```python
from build123d import *

# Parameters (mm, degrees)
SKETCH2_W           = 200
SKETCH2_H           = 95
BOSS_EXTRUDE1_DEPTH = 11
SKETCH3_W           = 200
SKETCH3_H           = 95
BOSS_EXTRUDE2_DEPTH = 2
SKETCH4_W           = 22
SKETCH4_H           = 35
SKETCH4_W_2         = 10
SKETCH4_H_2         = 26.5
SKETCH4_W_3         = 3
SKETCH4_H_3         = 8
SKETCH4_W_4         = 15
SKETCH4_H_4         = 15
BOSS_EXTRUDE3_DEPTH = 5
CUT_EXTRUDE1_DEPTH  = 7
SKETCH9_W           = 10
SKETCH9_H           = 3
BOSS_EXTRUDE4_DEPTH = 11
SKETCH7_W           = 220
SKETCH7_H           = 95
BOSS_EXTRUDE5_DEPTH = 2
FILLET1_R           = 2
FILLET2_R           = 2
SKETCH10_R          = 2.1
CUT_EXTRUDE2_DEPTH  = 6


with BuildPart() as part:
    # Sketch2 → Boss-Extrude1 (new body)
    with BuildSketch(Plane(origin=(0, 0, 0), x_dir=(1, 0, 0), z_dir=(0, 1, 0))):
        Rectangle(SKETCH2_W, SKETCH2_H)
        Polygon((21.5, 4.091136268), (21.5, 45), (93.5, 45), (93.5, -45), (21.5, -45), (21.5, -5.908863732), (10, -5.908863732), (10, -11), (-10, -31), (-71.5, -31), (-71.5, -41), (-93.5, -41), (-93.5, 41), (-71.5, 41), (-71.5, -16), (-10, -16), (-10, 8.5), (-19, 8.5), (-19, 43.5), (-10, 43.5), (-10, 46.5), (10, 46.5), (10, 43.5), (19, 43.5), (19, 8.5), (10, 8.5), (10, 4.091136268), align=None, mode=Mode.SUBTRACT)
    extrude(amount=BOSS_EXTRUDE1_DEPTH)

    # Sketch3 → Boss-Extrude2 (add)
    with BuildSketch(Plane.XZ):
        Rectangle(SKETCH3_W, SKETCH3_H)
    extrude(amount=BOSS_EXTRUDE2_DEPTH)

    # Sketch4 → Boss-Extrude3 (add)
    with BuildSketch(Plane(origin=(0, 0, 0), x_dir=(1, 0, 0), z_dir=(0, 1, 0))):
        with Locations((-82.5, 23.5)):
            Rectangle(SKETCH4_W, SKETCH4_H)
        with Locations((-0.04618168, 33.25)):
            Rectangle(SKETCH4_W_2, SKETCH4_H_2)
        with Locations((-92, -37)):
            Rectangle(SKETCH4_W_3, SKETCH4_H_3)
        with Locations((29, 37.5)):
            Rectangle(SKETCH4_W_4, SKETCH4_H_4)
        with Locations((86, 37.5)):
            Rectangle(SKETCH4_W_4, SKETCH4_H_4)
        with Locations((86, -37.5)):
            Rectangle(SKETCH4_W_4, SKETCH4_H_4)
        with Locations((29, -37.5)):
            Rectangle(SKETCH4_W_4, SKETCH4_H_4)
    extrude(amount=BOSS_EXTRUDE3_DEPTH)

    # Sketch5 → Cut-Extrude1 (cut)
    with BuildSketch(Plane.XY.offset(-46.5)):
        with BuildLine():
            Line((-2.94618168, 9.6), (2.85381832, 9.6))
            ThreePointArc((2.85381832, 9.6), (4.60381832, 7.85), (2.85381832, 6.1))
            Line((2.85381832, 6.1), (-2.94618168, 6.1))
            ThreePointArc((-2.94618168, 6.1), (-4.69618168, 7.85), (-2.94618168, 9.6))
        make_face()
    extrude(amount=-CUT_EXTRUDE1_DEPTH, mode=Mode.SUBTRACT)

    # Sketch9 → Boss-Extrude4 (add)
    with BuildSketch(Plane(origin=(0, 0, 0), x_dir=(1, 0, 0), z_dir=(0, 1, 0))):
        with Locations((-0.04618168, 18.5)):
            Rectangle(SKETCH9_W, SKETCH9_H)
    extrude(amount=BOSS_EXTRUDE4_DEPTH)

    # Sketch7 → Boss-Extrude5 (add)
    with BuildSketch(Plane.XZ.offset(2)):
        Rectangle(SKETCH7_W, SKETCH7_H)
    extrude(amount=-BOSS_EXTRUDE5_DEPTH)

    # Fillet1
    fillet1_edges = [part.edges().sort_by_distance(p)[0] for p in [
        (100, 0, 0),
        (-100, 0, 0),
    ]]
    fillet(fillet1_edges, radius=FILLET1_R)

    # Fillet2
    fillet2_edges = [part.edges().sort_by_distance(p)[0] for p in [
        (10, 5.5, -43.5),
        (-10, 5.5, -43.5),
        (-19, 5.5, -43.5),
        (-19, 5.5, -8.5),
        (-10, 5.5, -8.5),
        (-10, 5.5, 16),
        (-71.5, 5.5, 16),
        (-71.5, 5.5, 31),
        (-10, 5.5, 31),
        (10, 5.5, 11),
        (10, 5.5, 5.908863732),
        (21.5, 5.5, 5.908863732),
        (21.5, 5.5, -4.091136268),
        (10, 5.5, -4.091136268),
        (10, 5.5, -8.5),
        (19, 5.5, -8.5),
        (19, 5.5, -43.5),
    ]]
    fillet(fillet2_edges, radius=FILLET2_R)

    # Sketch10 → Cut-Extrude2 (cut)
    with BuildSketch(Plane(origin=(0, 11, 0), x_dir=(1, 0, 0), z_dir=(0, 1, 0))):
        with Locations(Location((-96, -43.5, 0), (0, 0, 270))):
            Circle(SKETCH10_R)
        with Locations(Location((-5, -43.5, 0), (0, 0, 270))):
            Circle(SKETCH10_R)
        with Locations(Location((5, -43.5, 0), (0, 0, 270))):
            Circle(SKETCH10_R)
        with Locations(Location((97, -43.5, 0), (0, 0, 270))):
            Circle(SKETCH10_R)
        with Locations(Location((97, 43.5, 0), (0, 0, 270))):
            Circle(SKETCH10_R)
        with Locations(Location((-26.428932188, 43.5, 0), (0, 0, 270))):
            Circle(SKETCH10_R)
        with Locations(Location((-36.428932188, 43.5, 0), (0, 0, 270))):
            Circle(SKETCH10_R)
        with Locations(Location((-96, 43.5, 0), (0, 0, 270))):
            Circle(SKETCH10_R)
    extrude(amount=-CUT_EXTRUDE2_DEPTH, mode=Mode.SUBTRACT)


solid = part.part
```
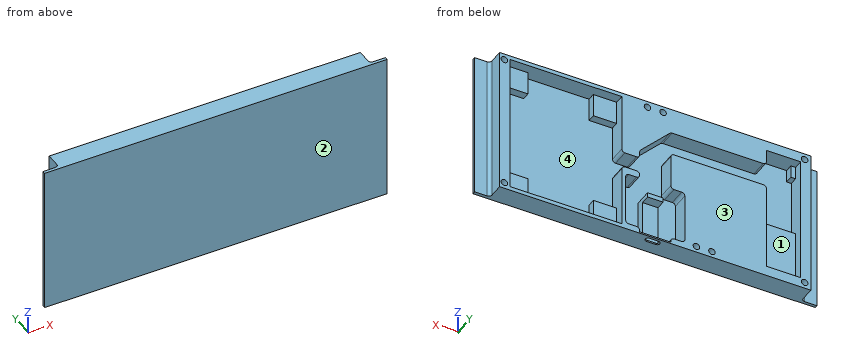
Read the model definition and answer for the solid it produces. Units are mm, in the model's axes. Face numbers are marked on the shaded views. A direction names the side the tool comes from. Coordinates: 2 decimals unless noted, no trailing zeros. Loops run counter-clockwise (first coordinate to the right, second up) from the corner with the lowest first, then second, coordinate; pieces in that order, holes last.
(1) A tool of negligible diameter and unlimited length cuts with its end or side. For the marked faces 1 and 2, from which of +Z, -Z, +X, -X, +Y, -Y can it reach the whole face along a straight path? Write none if from no direction.
Solution:
face 1: +Y
face 2: +Z, -Z, +X, -X, -Y
(2) Flat-ended cylindrical pins translate along their axes: pin 1 Ø1.5 at (y, z) = (3.5, 39) entering from +X; pin 2 Ø0.5 at (y, z) = (4.5, -46) entering from -X; pin 3 Ø3 at (x, z) = (0, -30) entering from +Y; pin 4 Ø4.5 at (x, z) = (-25.5, -43.5) entering from +Y. Find the tip coordinate at first contact, or state that the pin passes through.
Solution:
pin 1: stops at x = 100
pin 2: stops at x = -100
pin 3: stops at y = 5
pin 4: stops at y = 11
(3) Consider line 1 along X through (y, z) = (8, -21); line 2 along X through (y, z) = (8.9, 43.5); line 3 along X through (y, z) = (2.5, 9). Determine where each line is inside the solid, lowest interval first.
Solution:
line 1: x = -100 to -93.5, -71.5 to -19, 19 to 21.5, 93.5 to 100
line 2: x = -100 to -98.1, -93.9 to -7.1, -2.9 to 2.9, 7.1 to 21.5, 93.5 to 94.9, 99.1 to 100
line 3: x = -100 to -93.5, -71.5 to -10, 10 to 21.5, 93.5 to 100
(4) The part is cut by section B-B (x = -60.5). Determine the outline of the cut face in (y, z), and give its area (3 significant figures).
Solution:
outline: (-2, -47.5) - (11, -47.5) - (11, 16) - (0, 16) - (0, 31) - (11, 31) - (11, 47.5) - (-2, 47.5) - close
area: 1,070 mm2
(5) The mould has two halves that part along Z. Classify the marked faces 3 and 4: released by +Z, released by -Z, zero draft, split by the parting line, or undercut.
Solution:
face 3: zero draft
face 4: undercut
(6) The part is cut by section C-C (x = 70). Determine the outline of the cut face in (y, z).
Solution:
outline: (-2, -47.5) - (11, -47.5) - (11, -45) - (0, -45) - (0, 45) - (11, 45) - (11, 47.5) - (-2, 47.5) - close
(7) The part is cut by section A-A (x = -96). Determine the outline of the cut face in (y, z).
Solution:
outline: (-2, -47.5) - (11, -47.5) - (11, -45.6) - (5, -45.6) - (5, -41.4) - (11, -41.4) - (11, 41.4) - (5, 41.4) - (5, 45.6) - (11, 45.6) - (11, 47.5) - (-2, 47.5) - close
